```python
from build123d import *

# Parameters (mm, degrees)
SKETCH1_R           = 5
BOSS_EXTRUDE1_DEPTH = 10
SKETCH2_R           = 3.65
CUT_EXTRUDE1_DEPTH  = 10
CUT_EXTRUDE2_DEPTH  = 5
SKETCH5_R           = 5
SKETCH5_R_2         = 3.5
BOSS_EXTRUDE3_DEPTH = 0.5


with BuildPart() as part:
    # Sketch1 → Boss-Extrude1 (new body)
    with BuildSketch(Plane.XY):
        Circle(SKETCH1_R)
    extrude(amount=BOSS_EXTRUDE1_DEPTH)

    # Sketch2 → Cut-Extrude1 (cut)
    with BuildSketch(Plane.XY.offset(10)):
        Circle(SKETCH2_R)
    extrude(amount=-CUT_EXTRUDE1_DEPTH, mode=Mode.SUBTRACT)

    # Sketch4 → Cut-Extrude2 (cut)
    with BuildSketch(Plane(origin=(0, 0, 0), x_dir=(-1, 0, 0), z_dir=(0, 0, -1))):
        Polygon((0, 4.214656965), (-3.65, 2.107328483), (-3.65, -2.107328483), (0, -4.214656965), (3.65, -2.107328483), (3.65, 2.107328483), align=None)
    extrude(amount=-CUT_EXTRUDE2_DEPTH, mode=Mode.SUBTRACT)

    # Sketch5 → Boss-Extrude3 (add)
    with BuildSketch(Plane.XY.offset(10)):
        Circle(SKETCH5_R)
        Circle(SKETCH5_R_2, mode=Mode.SUBTRACT)
    extrude(amount=BOSS_EXTRUDE3_DEPTH)


solid = part.part
```
Can you work these out from the model? Positions are in its coordinate system, mm. A direction names the side the tool comes from. Round coordinates to 2 decimals unless told otherwise and drop trailing zeros. Order: outer loops, then holes, each group sorted by start corner. A loop starts at its lowest first (then second) coordinate and runs counter-clockwise, first axis right, second up.
(1) We'd pull the mould along Y, two halves only. Please class faces 3 (the face through (-3.3, -1.9, 5)), 4 (the face through (-1.08, -4.88, 5.18)), 5 (the face through (4, 0, 0)): +Y half, -Y half, draft (parallel to the pull), parting line (faces both ways), or undercut.
Results are:
face 3: undercut
face 4: parting line
face 5: draft
(2) If we section it at D-D (z = 7.75): Please give me the cut outline in (x, y), plus the area to 3 significant figures.
Results are:
outline: circle Ø10 at (0, 0); hole circle Ø7.3 at (0, 0)
area: 36.7 mm2
(3) If we section it at C-C (x = -0.25): Please give me the cut outline in (y, z), plus the area to 3 significant figures.
Results are:
outline: (-4.99, 0) - (-4.07, 0) - (-4.07, 5) - (-3.64, 5) - (-3.64, 10) - (-3.49, 10) - (-3.49, 10.5) - (-4.99, 10.5) - close; (3.49, 10) - (3.64, 10) - (3.64, 5) - (4.07, 5) - (4.07, 0) - (4.99, 0) - (4.99, 10.5) - (3.49, 10.5) - close
area: 24.3 mm2
(4) I'm going to push flat-ended pins straight in: pin 1 (1.5 mm diameter, centred on y = -1, z = 5, fed in from +X); pin 2 (3 mm diameter, centred on x = 2, z = 1.5, fed in from +Y). Where does each tip first touch, or does it pass through?
Results are:
pin 1: stops at x = 4.99
pin 2: stops at y = 4.97
(5) If we section it at A-A (z = 4.25): Please give me the cut outline in (x, y), plus the area to 3 significant figures.
Results are:
outline: circle Ø10 at (0, 0); hole (-3.65, -2.11) - (0, -4.21) - (3.65, -2.11) - (3.65, 2.11) - (0, 4.21) - (-3.65, 2.11) - close
area: 32.4 mm2
(6) If I drill on L1, parallel to Y at x = 0, z = 6.6; L2, parallel to Y at x = 0, z = 10.3; L3, parallel to X at y = 1.5, z = 8.25, over which ranges is the centre line in solid material (lowest first)?
Results are:
L1: y = -5 to -3.65, 3.65 to 5
L2: y = -5 to -3.5, 3.5 to 5
L3: x = -4.77 to -3.33, 3.33 to 4.77
(7) On a 3-axis mill with a long thin cutter (end or side, diameter ignored), from which of +Z, -Z, +X, -X, +Y, -Y can I reach the whole of each face in a straight line? I mean faces 1 (the face through (2.2, -3.3, 10.5)), 2 (the face through (0, -4, 5)). Say none if no direction works.
Results are:
face 1: +Z, +X, -X, +Y, -Y
face 2: -Z
